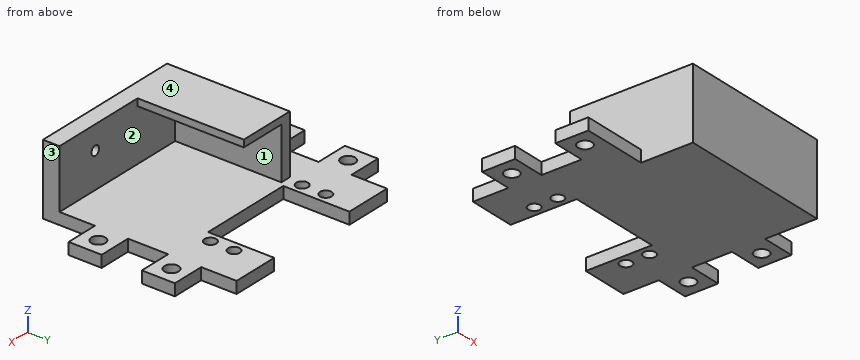
```python
from build123d import *

# Parameters (mm, degrees)
ESQUISSE1_W             = 80
ESQUISSE1_H             = 75
ESQUISSE1_W_2           = 40
ESQUISSE1_H_2           = 19
ESQUISSE1_W_3           = 14
ESQUISSE1_H_3           = 14
BOSS_EXTRU_1_DEPTH      = 5
ENL_V_MAT_EXTRU_1_REACH = 122.358
ESQUISSE2_R             = 3
ESQUISSE3_W             = 80
ESQUISSE3_H             = 7
BOSS_EXTRU_2_DEPTH      = 30
ENL_V_MAT_EXTRU_2_REACH = 125.94
ESQUISSE4_R             = 2.5
ENL_V_MAT_EXTRU_3_REACH = 125.94
ESQUISSE5_W             = 40
ESQUISSE5_H             = 9
ESQUISSE6_R             = 2
ENL_V_MAT_EXTRU_4_DEPTH = 4
ESQUISSE7_W             = 4.5
ESQUISSE7_H             = 45
BOSS_EXTRU_3_DEPTH      = 25
ESQUISSE8_W             = 3
ESQUISSE8_H             = 45
BOSS_EXTRU_4_DEPTH      = 20
ENL_V_MAT_EXTRU_5_REACH = 124.825
ESQUISSE9_W             = 14
ESQUISSE9_H             = 15
ENL_V_MAT_EXTRU_9_REACH = 125.94
ESQUISSE11_W            = 14
ESQUISSE11_H            = 7


with BuildPart() as part:
    # Esquisse1 → Boss.-Extru.1 (new body)
    # profile 1 of 5: a face of its own
    with BuildSketch(Plane.XY):
        with Locations((40, 37.5)):
            Rectangle(ESQUISSE1_W, ESQUISSE1_H)
        with Locations((40, 56.5)):
            Rectangle(ESQUISSE1_W_2, ESQUISSE1_H_2, mode=Mode.SUBTRACT)
    # profile 2 of 5: a face of its own
    with BuildSketch(Plane.XY):
        with Locations((-7, 53)):
            Rectangle(ESQUISSE1_W_3, ESQUISSE1_H_3)
    # profile 3 of 5: a face of its own
    with BuildSketch(Plane.XY):
        with Locations((-7, 22)):
            Rectangle(ESQUISSE1_W_3, ESQUISSE1_H_3)
    # profile 4 of 5: a face of its own
    with BuildSketch(Plane.XY):
        with Locations((87, 53)):
            Rectangle(ESQUISSE1_W_3, ESQUISSE1_H_3)
    # profile 5 of 5: a face of its own
    with BuildSketch(Plane.XY):
        with Locations((87, 22)):
            Rectangle(ESQUISSE1_W_3, ESQUISSE1_H_3)
    extrude(amount=BOSS_EXTRU_1_DEPTH)

    # Esquisse2 → Enlèv. mat.-Extru.1 (cut, up to next)
    with BuildSketch(Plane.XY.offset(5), mode=Mode.PRIVATE) as enl_v_mat_extru_1_sk1:
        with Locations((-7, 53)):
            Circle(ESQUISSE2_R)
    enl_v_mat_extru_1_tool1 = extrude(enl_v_mat_extru_1_sk1.sketch, amount=-ENL_V_MAT_EXTRU_1_REACH, mode=Mode.PRIVATE) & part.part
    # Esquisse2 → Enlèv. mat.-Extru.1 (cut, up to next)
    with BuildSketch(Plane.XY.offset(5), mode=Mode.PRIVATE) as enl_v_mat_extru_1_sk2:
        with Locations((-7, 22)):
            Circle(ESQUISSE2_R)
    enl_v_mat_extru_1_tool2 = extrude(enl_v_mat_extru_1_sk2.sketch, amount=-ENL_V_MAT_EXTRU_1_REACH, mode=Mode.PRIVATE) & part.part
    # Esquisse2 → Enlèv. mat.-Extru.1 (cut, up to next)
    with BuildSketch(Plane.XY.offset(5), mode=Mode.PRIVATE) as enl_v_mat_extru_1_sk3:
        with Locations((87, 22)):
            Circle(ESQUISSE2_R)
    enl_v_mat_extru_1_tool3 = extrude(enl_v_mat_extru_1_sk3.sketch, amount=-ENL_V_MAT_EXTRU_1_REACH, mode=Mode.PRIVATE) & part.part
    # Esquisse2 → Enlèv. mat.-Extru.1 (cut, up to next)
    with BuildSketch(Plane.XY.offset(5), mode=Mode.PRIVATE) as enl_v_mat_extru_1_sk4:
        with Locations((87, 53)):
            Circle(ESQUISSE2_R)
    enl_v_mat_extru_1_tool4 = extrude(enl_v_mat_extru_1_sk4.sketch, amount=-ENL_V_MAT_EXTRU_1_REACH, mode=Mode.PRIVATE) & part.part
    add(enl_v_mat_extru_1_tool1.solids().sort_by_distance((-7, 53, 5))[0], mode=Mode.SUBTRACT)
    add(enl_v_mat_extru_1_tool2.solids().sort_by_distance((-7, 22, 5))[0], mode=Mode.SUBTRACT)
    add(enl_v_mat_extru_1_tool3.solids().sort_by_distance((87, 22, 5))[0], mode=Mode.SUBTRACT)
    add(enl_v_mat_extru_1_tool4.solids().sort_by_distance((87, 53, 5))[0], mode=Mode.SUBTRACT)

    # Esquisse3 → Boss.-Extru.2 (add)
    with BuildSketch(Plane.XY):
        with Locations((40, -3.5)):
            Rectangle(ESQUISSE3_W, ESQUISSE3_H)
    extrude(amount=BOSS_EXTRU_2_DEPTH)

    # Esquisse4 → Enlèv. mat.-Extru.2 (cut, up to next)
    with BuildSketch(Plane(origin=(0, 0, 0), x_dir=(-1, 0, 0), z_dir=(0, 0, -1)), mode=Mode.PRIVATE) as enl_v_mat_extru_2_sk1:
        with Locations((-64.4, 61.5)):
            Circle(ESQUISSE4_R)
    enl_v_mat_extru_2_tool1 = extrude(enl_v_mat_extru_2_sk1.sketch, amount=-ENL_V_MAT_EXTRU_2_REACH, mode=Mode.PRIVATE) & part.part
    # Esquisse4 → Enlèv. mat.-Extru.2 (cut, up to next)
    with BuildSketch(Plane(origin=(0, 0, 0), x_dir=(-1, 0, 0), z_dir=(0, 0, -1)), mode=Mode.PRIVATE) as enl_v_mat_extru_2_sk2:
        with Locations(Location((-15.6, 61.5, 0), (0, 0, 180))):
            Circle(ESQUISSE4_R)
    enl_v_mat_extru_2_tool2 = extrude(enl_v_mat_extru_2_sk2.sketch, amount=-ENL_V_MAT_EXTRU_2_REACH, mode=Mode.PRIVATE) & part.part
    # Esquisse4 → Enlèv. mat.-Extru.2 (cut, up to next)
    with BuildSketch(Plane(origin=(0, 0, 0), x_dir=(-1, 0, 0), z_dir=(0, 0, -1)), mode=Mode.PRIVATE) as enl_v_mat_extru_2_sk3:
        with Locations((-15.6, 51.5)):
            Circle(ESQUISSE4_R)
    enl_v_mat_extru_2_tool3 = extrude(enl_v_mat_extru_2_sk3.sketch, amount=-ENL_V_MAT_EXTRU_2_REACH, mode=Mode.PRIVATE) & part.part
    # Esquisse4 → Enlèv. mat.-Extru.2 (cut, up to next)
    with BuildSketch(Plane(origin=(0, 0, 0), x_dir=(-1, 0, 0), z_dir=(0, 0, -1)), mode=Mode.PRIVATE) as enl_v_mat_extru_2_sk4:
        with Locations(Location((-64.4, 51.5, 0), (0, 0, 180))):
            Circle(ESQUISSE4_R)
    enl_v_mat_extru_2_tool4 = extrude(enl_v_mat_extru_2_sk4.sketch, amount=-ENL_V_MAT_EXTRU_2_REACH, mode=Mode.PRIVATE) & part.part
    add(enl_v_mat_extru_2_tool1.solids().sort_by_distance((64.4, 61.5, 0))[0], mode=Mode.SUBTRACT)
    add(enl_v_mat_extru_2_tool2.solids().sort_by_distance((15.6, 61.5, 0))[0], mode=Mode.SUBTRACT)
    add(enl_v_mat_extru_2_tool3.solids().sort_by_distance((15.6, 51.5, 0))[0], mode=Mode.SUBTRACT)
    add(enl_v_mat_extru_2_tool4.solids().sort_by_distance((64.4, 51.5, 0))[0], mode=Mode.SUBTRACT)

    # Esquisse5 → Enlèv. mat.-Extru.3 (cut, up to next)
    with BuildSketch(Plane(origin=(0, 0, 0), x_dir=(-1, 0, 0), z_dir=(0, 0, -1)), mode=Mode.PRIVATE) as enl_v_mat_extru_3_sk1:
        with Locations((-40, 70.5)):
            Rectangle(ESQUISSE5_W, ESQUISSE5_H)
    enl_v_mat_extru_3_tool1 = extrude(enl_v_mat_extru_3_sk1.sketch, amount=-ENL_V_MAT_EXTRU_3_REACH, mode=Mode.PRIVATE) & part.part
    add(enl_v_mat_extru_3_tool1.solids().sort_by_distance((40, 70.5, 0))[0], mode=Mode.SUBTRACT)

    # Esquisse6 → Enlèv. mat.-Extru.4 (cut)
    with BuildSketch(Plane(origin=(0, 0, 0), x_dir=(1, 0, 0), z_dir=(0, 1, 0))):
        with Locations(Location((61, -20, 0), (0, 0, 270))):
            Circle(ESQUISSE6_R)
    extrude(amount=-ENL_V_MAT_EXTRU_4_DEPTH, mode=Mode.SUBTRACT)

    # Esquisse7 → Boss.-Extru.3 (add)
    with BuildSketch(Plane.XY.offset(5)):
        with Locations((16.25, 22.5)):
            Rectangle(ESQUISSE7_W, ESQUISSE7_H)
    extrude(amount=BOSS_EXTRU_3_DEPTH)

    # Esquisse8 → Boss.-Extru.4 (add)
    with BuildSketch(Plane(origin=(18.5, 0, 0), x_dir=(0, 0, -1), z_dir=(1, 0, 0))):
        with Locations((-28.5, 22.5)):
            Rectangle(ESQUISSE8_W, ESQUISSE8_H)
    extrude(amount=BOSS_EXTRU_4_DEPTH)

    # Esquisse9 → Enlèv. mat.-Extru.5 (cut, up to next)
    with BuildSketch(Plane.XY.offset(5), mode=Mode.PRIVATE) as enl_v_mat_extru_5_sk1:
        with Locations((7, 7.5)):
            Rectangle(ESQUISSE9_W, ESQUISSE9_H)
    enl_v_mat_extru_5_tool1 = extrude(enl_v_mat_extru_5_sk1.sketch, amount=-ENL_V_MAT_EXTRU_5_REACH, mode=Mode.PRIVATE) & part.part
    add(enl_v_mat_extru_5_tool1.solids().sort_by_distance((7, 7.5, 5))[0], mode=Mode.SUBTRACT)

    # Esquisse11 → Enlèv. mat.-Extru.9 (cut, up to next)
    with BuildSketch(Plane.XY.offset(30), mode=Mode.PRIVATE) as enl_v_mat_extru_9_sk1:
        with Locations((7, -3.5)):
            Rectangle(ESQUISSE11_W, ESQUISSE11_H)
    enl_v_mat_extru_9_tool1 = extrude(enl_v_mat_extru_9_sk1.sketch, amount=-ENL_V_MAT_EXTRU_9_REACH, mode=Mode.PRIVATE) & part.part
    add(enl_v_mat_extru_9_tool1.solids().sort_by_distance((7, -3.5, 30))[0], mode=Mode.SUBTRACT)


solid = part.part
```
Geometry check sheet. Reference: the model listing, model coordinates, mm. Face numbers are marked on the shaded views. Coordinates: 2 decimals unless noted, no trailing zeros. Loops run counter-clockwise (first coordinate to the right, second up) from the corner with the lowest first, then second, coordinate; pieces in that order, holes last.
Item 1: Go/stop test with flat-tipped pins: pin 1 Ø12 at (x, z) = (30.5, 19.5) entering from +Y; pin 2 Ø3 at (x, y) = (64.4, 61.5) entering from +Z; pin 3 Ø4 at (x, z) = (85, 1.5) entering from +Y; pin 4 Ø11 at (y, z) = (26, 21) entering from +X. Record where each tip stops, or that it passes through.
Item 2: Sectioned sample at D-D, the plane x = 87. Record the boundary of the cut face in (y, z).
Item 3: Sectioned sample at C-C, the plane x = 64.4. Record the boundary of the cut face in (y, z), then the cut area to 3 significant figures.
Item 4: Sectioned sample at B-B, the plane z = 3.75. Count the separate pieces of the cut face and the enclosed holes in it, then the cut area to 3 significant figures.
Item 5: Thickness scan on line 1 (Y direction, x = 64.4, z = 2.5); line 2 (Y direction, x = 87, z = 3.1); line 3 (Z direction, x = 25, y = 46). Record the ranges inside material, lowest first.
Item 6: Release check for a two-part mould opening along Z. For the marked faces 1, 2, 3 and 4 record: released by +Z, released by -Z, zero draft, split by the parting line, or undercut.
Item 7: Sectioned sample at A-A, the plane y = 61.5. Record the boundary of the cut face in (x, z).
Check result:
1. pin 1: stops at y = 0
1. pin 2: passes through
1. pin 3: stops at y = 60
1. pin 4: stops at x = 18.5
2. outline: (15, 0) - (19, 0) - (19, 5) - (15, 5) - close; (25, 0) - (29, 0) - (29, 5) - (25, 5) - close; (46, 0) - (50, 0) - (50, 5) - (46, 5) - close; (56, 0) - (60, 0) - (60, 5) - (56, 5) - close
3. outline: (-7, 0) - (49, 0) - (49, 5) - (0, 5) - (0, 30) - (-7, 30) - close; (54, 0) - (59, 0) - (59, 5) - (54, 5) - close; (64, 0) - (75, 0) - (75, 5) - (64, 5) - close
3. area: 535 mm2
4. separate pieces: 1
4. enclosed holes: 8
4. area: 5,720 mm2
5. line 1: y = -7 to 49, 54 to 59, 64 to 75
5. line 2: y = 15 to 19, 25 to 29, 46 to 50, 56 to 60
5. line 3: z = 0 to 5
6. face 1: undercut
6. face 2: undercut
6. face 3: zero draft
6. face 4: released by +Z
7. outline: (0, 0) - (13.1, 0) - (13.1, 5) - (0, 5) - close; (18.1, 0) - (20, 0) - (20, 5) - (18.1, 5) - close; (60, 0) - (61.9, 0) - (61.9, 5) - (60, 5) - close; (66.9, 0) - (80, 0) - (80, 5) - (66.9, 5) - close
